Input: part model. Units: mm. Frame: model coordinates. Round coordinates to 2 decimals unless told otherwise and drop trailing zeros. Write each loop counter-clockwise with the first axis right and the second up, starting at its lowest first coordinate (ties: lowest second). Pieces come first, ordered by that corner, then holes. Notation, with made-up numbers: (77, 55.5) - (119, 55.5) arc R16 cw to (119, 79.5) - close; hole circle Ø11 at (-9.5, 45.25). An arc over 180 degrees is marked (long way). Use one line per item in the form item = value.
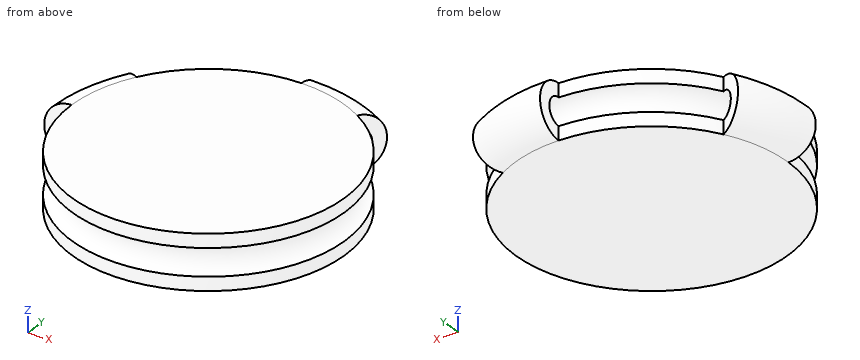
```python
from build123d import *

# Parameters (mm, degrees)
ESQUISSE1_R                             = 10
BOSS_EXTRU_1_DEPTH                      = 2
ESQUISSE4_R                             = 2
R_VOLUTION1_ANGLE                       = 120
ESQUISSE2_R                             = 1
ENL_VEMENT_DE_MATI_RE_R_VOLUTION2_ANGLE = 60


with BuildPart() as part:
    # Esquisse1 → Boss.-Extru.1 (new body, symmetric)
    with BuildSketch(Plane.XY):
        Circle(ESQUISSE1_R)
    extrude(amount=BOSS_EXTRU_1_DEPTH, both=True)

    # Esquisse4 → Révolution1 (revolve)
    with BuildSketch(Plane(origin=(0, 0, 0), x_dir=(1, 0, 0), z_dir=(0, 1, 0))):
        with Locations((-10, 0)):
            Circle(ESQUISSE4_R)
    revolve(axis=Axis((0, 0, 2), (0, 0, -1)), revolution_arc=R_VOLUTION1_ANGLE)

    # Esquisse2 → Enlèvement de matière-Révolution1 (revolve, cut)
    with BuildSketch(Plane(origin=(0, 0, 0), x_dir=(0, 0, -1), z_dir=(1, 0, 0))):
        with Locations((0, 10)):
            Circle(ESQUISSE2_R)
    revolve(axis=Axis((0, 0, -8.634448203), (0, 0, 1)), mode=Mode.SUBTRACT)

    # Esquisse6 → Enlèvement de matière-Révolution2 (revolve, cut)
    with BuildSketch(Plane(origin=(0, 0, 0), x_dir=(0, 0, -1), z_dir=(1, 0, 0))):
        with BuildLine():
            Line((-2, 10), (-1, 10))
            ThreePointArc((-1, 10), (0, 11), (1, 10))
            Line((1, 10), (2, 10))
            ThreePointArc((2, 10), (0, 12), (-2, 10))
        make_face()
    revolve(axis=Axis((0, 0, 0), (0, 0, 1)), revolution_arc=ENL_VEMENT_DE_MATI_RE_R_VOLUTION2_ANGLE, mode=Mode.SUBTRACT)


solid = part.part
```
(1) Cut plane A-A on z = -0.2. Output: boundary loops of the cut face in (x, y).
Derived:
outline = (-11.99, 0) - (-10.98, 0) arc R10.98 cw to (-9.51, 5.49) - (-10.38, 5.99) arc R11.99 ccw to start; circle Ø18.04 at (0, 0); (0, 10.98) arc R10.98 cw to (5.49, 9.51) - (5.99, 10.38) arc R11.99 ccw to (0, 11.99) - close
(2) Material intervals for L1, parallel to X at y = 4.5, z = 0; L2, parallel to Y at x = 5.25, z = 0; L3, parallel to Y at x = 4.75, z = 0.2, sorted ascending.
Derived:
L1 = -11.12 to -10.04, -7.79 to 7.79
L2 = -7.31 to 7.31, 9.67 to 10.79
L3 = -7.67 to 7.67, 9.9 to 11.01
(3) First-contact query: pin 1 Ø1 at (x, z) = (-11, -1) entering from -Y; pin 2 Ø2 at (y, z) = (11, 0) entering from -X; pin 3 Ø1.5 at (y, z) = (-1.5, -1) entering from +X. Flat tips, straight axial feed; report the tip coordinate or a pass-through.
Derived:
pin_1 = 0
pin_2 = 0
pin_3 = 9.97
